Model file for the job. Use its own axes, mm. Face numbers are marked on the shaded views. A direction names the side the tool comes from. Coordinates: 2 decimals unless noted, no trailing zeros. Order: outer loops, then holes, each group sorted by start corner. A loop starts at its lowest first (then second) coordinate and runs counter-clockwise, first axis right, second up. Notation, with made-up numbers: (20.5, 46.25) -> (24.5, 46.25) arc R15 ccw to (24.5, 53.25) -> close; hole circle Ø7 at (-1, -10). An arc over 180 degrees is marked (long way). Use CSV: the item, a comma, the result in double quotes. Start each with the question number.
(1) Tool access for the marked faces 1 and 2: list every direction of +Z, -Z, +X, -X, +Y, -Y with a clear straight run to the whole face (end or side of a thin tool).
(2) Cut at A-A on x = 0. Write the cut outline in (y, z).
(3) Pull direction Y, two halves, no side cores. Call the marked faces 3, 4 and 5: pulls with the +Y half, pulls with the -Y half, needs draft (parallel to the pull), parting line crosses it, or undercut.
(4) Probe L1, parallel to Z at x = 0, y = 2; L2, parallel to Y at x = 0, z = -3.8; L3, parallel to X at y = 14.5, z = -3. List the from-to ranges inside material, lowest first.
(5) Cut at B-B on y = -2. Write the cut outline in (x, z).
(6) Pin check, flat tips, straight feed: pin 1 Ø1 at (x, y) = (-3, 0.5) entering from +Z; pin 2 Ø1.5 at (y, z) = (14, -1.5) entering from -X; pin 3 Ø3 at (y, z) = (13, 4) entering from +X. Stop position of each tip, or through.
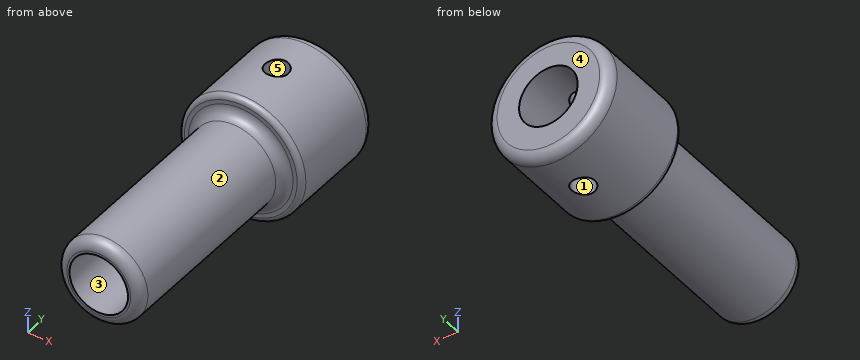
```python
from build123d import *

# Parameters (mm, degrees)
SKETCH2_R               = 1.1303
CUT_EXTRUDE1_DEPTH      = 10
CUT_EXTRUDE1_DEPTH_BACK = 10


with BuildPart() as part:
    # Sketch1 → Revolve1 (revolve)
    with BuildSketch(Plane.XY):
        with BuildLine():
            Line((2.85, 19.132875201), (5, 19.132875201))
            ThreePointArc((5, 19.132875201), (5.707106781, 18.839981982), (6, 18.132875201))
            Line((6, 18.132875201), (6, 9.632875201))
            ThreePointArc((6, 9.632875201), (5.853553391, 9.27932181), (5.5, 9.132875201))
            Line((5.5, 9.132875201), (5.1, 9.132875201))
            ThreePointArc((5.1, 9.132875201), (4.392893219, 8.839981982), (4.1, 8.132875201))
            Line((4.1, 8.132875201), (4.1, -9.867124799))
            ThreePointArc((4.1, -9.867124799), (3.807106781, -10.57423158), (3.1, -10.867124799))
            Line((3.1, -10.867124799), (2.85, -10.867124799))
            Line((2.85, -10.867124799), (2.85, 19.132875201))
        make_face()
    revolve(axis=Axis((0, 27.883391117, 0), (0, -1, 0)))

    # Sketch2 → Cut-Extrude1 (cut, two sides)
    with BuildSketch(Plane.XY) as cut_extrude1_sk:
        with Locations((0, 14.207956768)):
            Circle(SKETCH2_R)
    extrude(amount=CUT_EXTRUDE1_DEPTH, mode=Mode.SUBTRACT)
    extrude(cut_extrude1_sk.sketch, amount=-CUT_EXTRUDE1_DEPTH_BACK, mode=Mode.SUBTRACT)


solid = part.part
```
Outcome:
1,face 1,"+Z, -Z"
1,face 2,"-Y"
2,outline,"(-10.87, -3.1) arc R1 ccw to (-9.87, -4.1) -> (8.13, -4.1) arc R1 cw to (9.13, -5.1) -> (9.13, -5.5) arc R0.5 ccw to (9.63, -6) -> (13.08, -6) -> (13.08, -2.85) -> (-10.87, -2.85) -> close; (-10.87, 2.85) -> (13.08, 2.85) -> (13.08, 6) -> (9.63, 6) arc R0.5 ccw to (9.13, 5.5) -> (9.13, 5.1) arc R1 cw to (8.13, 4.1) -> (-9.87, 4.1) arc R1 ccw to (-10.87, 3.1) -> close; (15.34, -6) -> (18.13, -6) arc R1 ccw to (19.13, -5) -> (19.13, -2.85) -> (15.34, -2.85) -> close; (15.34, 2.85) -> (19.13, 2.85) -> (19.13, 5) arc R1 ccw to (18.13, 6) -> (15.34, 6) -> close"
3,face 3,"needs draft"
3,face 4,"pulls with the +Y half"
3,face 5,"undercut"
4,L1,"-4.1 to -2.85, 2.85 to 4.1"
4,L2,"-10.58 to 13.08, 15.34 to 19.13"
4,L3,"-5.2 to -1.09, 1.09 to 5.2"
5,outline,"circle Ø8.2 at (0, 0); hole circle Ø5.7 at (0, 0)"
6,pin 1,"z = 3.25"
6,pin 2,"x = -5.95"
6,pin 3,"x = 5.45"
